Read the model definition and answer for the solid it produces. Units are mm, in the model's axes. A direction names the side the tool comes from. Round coordinates to 2 decimals unless told otherwise and drop trailing zeros. Loops run counter-clockwise (first coordinate to the right, second up) from the corner with the lowest first, then second, coordinate; pieces in that order, holes last. Notation, with made-up numbers: (48.5, 8.5) - (56.5, 8.5) arc R24 ccw to (56.5, 42.5) - close; hole circle Ø11 at (-18, 27.25). An arc over 180 degrees is marked (long way). Answer as CSV lines item,"result".
```python
from build123d import *

# Parameters (mm, degrees)
F0_R     = 18.25
F1_DEPTH = 203
F2_R     = 5
F3_DEPTH = 10
F4_R     = 5
F5_SIZE  = 8


with BuildPart() as f1:
    # F0 (on Front) → F1 (new body)
    with BuildSketch(Plane.XZ):
        Circle(F0_R)
    extrude(amount=F1_DEPTH)

    # F2 (on Front) → F3 (join)
    with BuildSketch(Plane.XZ):
        Circle(F2_R)
    extrude(amount=-F3_DEPTH)

    # F4
    f4_edges = [f1.edges().sort_by_distance(p)[0] for p in [
        (-5, 10, 0),
    ]]
    fillet(f4_edges, radius=F4_R)

    # F5
    f5_edges = [f1.edges().sort_by_distance(p)[0] for p in [
        (-18.25, 0, 0),
    ]]
    chamfer(f5_edges, length=F5_SIZE)


solid = f1.part
```
1) Find the intervals of material crossed by line 1 (Y direction, x = 7, z = 4); line 2 (Z direction, x = 1, y = -163.5); line 3 (X direction, y = -93, z = 0.5), in increasing order.
Entries:
line 1,"y = -203 to 0"
line 2,"z = -18.22 to 18.22"
line 3,"x = -18.24 to 18.24"
2) A cutting plane is placed at B-B, the plane x = 0. Determine the outline of the cut face in (y, z).
Entries:
outline,"(-203, -18.25) - (-8, -18.25) - (0, -10.25) - (0, -5) - (5, -5) arc R5 ccw to (5, 5) - (0, 5) - (0, 10.25) - (-8, 18.25) - (-203, 18.25) - close"
3) A cutting plane is placed at C-C, the plane y = -187.5. Determine the outline of the cut face in (x, z).
Entries:
outline,"circle Ø36.5 at (0, 0)"
4) A tool of negligible diameter and unlimited length cuts with its end or side. For faces 1 (the face through (-3.956, -104.135, -17.816)), 2 (the face through (-1.08, 2.46, -4.88)), from which of +Z, -Z, +X, -X, +Y, -Y can it reach the whole face along a straight path? Write none if from no direction.
Entries:
face 1,"+Y, -Y"
face 2,"+Y"
5) A cutting plane is placed at A-A, the plane z = 0. Determine the outline of the cut face in (x, y).
Entries:
outline,"(-18.25, -203) - (18.25, -203) - (18.25, -8) - (10.25, 0) - (5, 0) - (5, 5) arc R5 ccw to (-5, 5) - (-5, 0) - (-10.25, 0) - (-18.25, -8) - close"
6) Each of these flat-tipped pins is pushed along its axis until it touches: P1, Ø3, axis at x = -12, y = -63, coming from the +Z side; P2, Ø5, axis at y = -65.5, z = 7, coming from the +X side; P3, Ø6, axis at x = -12.5, y = -21.5, coming from the -Z side. Where does it stop, or does it pass through?
Entries:
P1,"stops at z = 14.93"
P2,"stops at x = 17.69"
P3,"stops at z = -15.58"
